Source: CAD feature listing. Evaluate the final solid. Frame: model axes, mm. A direction names the side the tool comes from. Round coordinates to 2 decimals unless told otherwise and drop trailing zeros. Order: outer loops, then holes, each group sorted by start corner. A loop starts at its lowest first (then second) coordinate and runs counter-clockwise, first axis right, second up. Notation, with made-up numbers: (-11, -13.5) -> (-1, -13.5) arc R26 ccw to (-1, 24.5) -> close; hole circle Ø6 at (64, 12.25). An arc over 180 degrees is marked (long way). Answer as CSV lines item,"result". Start each with the question number.
(1) Set-up query: faces 4 (the flat face through (87.5, -4, -5)), 5 (the flat face through (-52.5, -4, -5)), 6 (the flat face through (-121, -4, 60)). Return all of +Z, -Z, +X, -X, +Y, -Y with unobstructed straight access to the full face (end or side cutting, diameter ignored); none if empty.
(2) Line query: line 1 along X through (y, z) = (-4.75, -4); line 2 along Z through (x, y) = (106, -6); line 3 along X through (y, z) = (-5.25, 53.5). Output: solid intervals per line, ascending. Write a range as from..to.
(3) Section query B-B (x = -45.5). Output: boundary loops of the cut face in (y, z), plus the area to 3 significant figures.
(4) Section query C-C (z = 47). Output: boundary loops of the cut face in (x, y).
(5) Pull-direction query (X, two-part tool) for faces 1 (the flat face through (-107, -4, 0)), 2 (the flat face through (-87.5, -4, -4)), 3 (the flat face through (52.5, -4, -4)); classes: +X half, -X half, draft (parallel to the pull), parting line (faces both ways), or undercut.
(6) Contact query for flat-ended pins moving along their axis: P1, Ø2.5, axis at y = -3.5, z = 48.5, coming from the +X side; P2, Ø4.5, axis at y = -6.5, z = -4, coming from the +X side; P3, Ø4, axis at y = -8, z = 38, coming from the -X side. Output: stop coordinate, or through.
(7) Section query A-A (y = -2.5). Output: boundary loops of the cut face in (x, z).
```python
from build123d import *

# Parameters (mm, degrees)
F1_DEPTH = 9


with BuildPart() as f1:
    # F0 (on Front) → F1 (new body)
    with BuildSketch(Plane.XZ):
        Polygon((0, 90), (-125, 90), (-125, 60), (-116, 60), (-116, 30), (-125, 30), (-125, 0), (-116, 0), (-87.5, 0), (-87.5, -9), (-52.5, -9), (-52.5, 0), (-17.5, 0), (-17.5, -9), (0, -9), (17.5, -9), (17.5, 0), (52.5, 0), (52.5, -9), (87.5, -9), (87.5, 0), (125, 0), (125, 30), (116, 30), (116, 60), (125, 60), (125, 90), align=None)
    extrude(amount=F1_DEPTH)


solid = f1.part
```
Answer block:
1,face 4,"-Z, +X, +Y, -Y"
1,face 5,"-Z, +Y, -Y"
1,face 6,"-X, +Y, -Y"
2,line 1,"-87.5..-52.5, -17.5..17.5, 52.5..87.5"
2,line 2,"0..90"
2,line 3,"-116..116"
3,outline,"(-9, 0) -> (0, 0) -> (0, 90) -> (-9, 90) -> close"
3,area,"810 mm2"
4,outline,"(-116, -9) -> (116, -9) -> (116, 0) -> (-116, 0) -> close"
5,face 1,"draft"
5,face 2,"-X half"
5,face 3,"undercut"
6,P1,"x = 116"
6,P2,"x = 87.5"
6,P3,"x = -116"
7,outline,"(-125, 0) -> (-87.5, 0) -> (-87.5, -9) -> (-52.5, -9) -> (-52.5, 0) -> (-17.5, 0) -> (-17.5, -9) -> (17.5, -9) -> (17.5, 0) -> (52.5, 0) -> (52.5, -9) -> (87.5, -9) -> (87.5, 0) -> (125, 0) -> (125, 30) -> (116, 30) -> (116, 60) -> (125, 60) -> (125, 90) -> (-125, 90) -> (-125, 60) -> (-116, 60) -> (-116, 30) -> (-125, 30) -> close"
